For this review, take the finished solid that the model builds, in its own axes (mm). A direction names the side the tool comes from. Give positions to 0.01 mm unless a question says otherwise; leave off trailing zeros. Write each loop counter-clockwise with the first axis right and the second up, starting at its lowest first coordinate (ties: lowest second). Pieces come first, ordered by that corner, then holes. Notation, with made-up numbers: (69.5, -16.75) -> (126.5, -16.75) arc R28 ccw to (126.5, 14.25) -> close; hole circle Ø7 at (45, 7.5). An arc over 180 degrees is marked (long way). Write item = value, one per line.
```python
from build123d import *

# Parameters (mm, degrees)
F0_W     = 76.2
F0_H     = 76.2
F1_DEPTH = 76.2
F2_R     = 11.2668024736
F3_DEPTH = 76.201
F4_W     = 32.2091430426
F4_H     = 35.9837710857
F5_DEPTH = 76.201
F6_R     = 5.08
F7_R     = 5.08


with BuildPart() as f1:
    # F0 (on Top) → F1 (new body)
    with BuildSketch(Plane.XY):
        with Locations((38.1, 38.1)):
            Rectangle(F0_W, F0_H)
    extrude(amount=F1_DEPTH)

    # F2 (on face) → F3 (cut, through all)
    with BuildSketch(Plane.XY.offset(76.2)):
        with Locations((35.9600186348, 40.4836237431)):
            Circle(F2_R)
    extrude(amount=-F3_DEPTH, mode=Mode.SUBTRACT)

    # F4 (on face) → F5 (cut, through all)
    with BuildSketch(Plane.YZ.offset(76.2)):
        with Locations((35.8842462301, 41.1003679037)):
            Rectangle(F4_W, F4_H)
    extrude(amount=-F5_DEPTH, mode=Mode.SUBTRACT)

    # F6
    f6_edges = [f1.edges().sort_by_distance(p)[0] for p in [
        (38.1, 0, 76.2),
        (76.2, 38.1, 76.2),
        (38.1, 76.2, 76.2),
        (0, 38.1, 76.2),
        (0, 0, 38.1),
        (76.2, 0, 38.1),
        (38.1, 0, 0),
        (76.2, 38.1, 0),
        (76.2, 35.884246, 23.108482),
        (76.2, 51.988818, 41.100368),
        (76.2, 76.2, 38.1),
        (76.2, 19.779675, 41.100368),
        (76.2, 35.884246, 59.092253),
        (0, 76.2, 38.1),
        (38.1, 76.2, 0),
        (0, 38.1, 0),
        (24.693216, 40.483624, 0),
    ]]
    fillet(f6_edges, radius=F6_R)

    # F7
    f7_edges = [f1.edges().sort_by_distance(p)[0] for p in [
        (38.1, 5.08, 76.2),
        (5.08, 38.1, 76.2),
        (71.12, 38.1, 76.2),
        (38.1, 71.12, 76.2),
        (24.693216, 40.483624, 76.2),
        (0, 38.1, 71.12),
        (0, 71.12, 38.1),
        (0, 5.08, 38.1),
        (0, 38.1, 5.08),
        (0, 51.988818, 41.100368),
        (0, 35.884246, 59.092253),
        (0, 19.779675, 41.100368),
        (0, 35.884246, 23.108482),
    ]]
    fillet(f7_edges, radius=F7_R)


solid = f1.part
```
(1) Take a section at B-B (x = 18). Write out the cut boundary in (y, z), plus the area to 3 significant figures.
Answers below:
outline = (0, 5.08) arc R5.08 ccw to (5.08, 0) -> (71.12, 0) arc R5.08 ccw to (76.2, 5.08) -> (76.2, 71.12) arc R5.08 ccw to (71.12, 76.2) -> (5.08, 76.2) arc R5.08 ccw to (0, 71.12) -> close; hole (19.78, 23.11) -> (51.99, 23.11) -> (51.99, 59.09) -> (19.78, 59.09) -> close
area = 4,630 mm^2
(2) For pin 1 (13.5 mm diameter, centred on x = 35.96, y = 40.48, fed in from -Z), flat-tipped, find the tip position at first contact; note if it passes through.
Answers below:
pin_1 = through
(3) Take a section at C-C (z = 60.5). Write out the cut boundary in (x, y), plus the area to 3 significant figures.
Answers below:
outline = (0, 5.08) arc R5.08 ccw to (5.08, 0) -> (71.12, 0) arc R5.08 ccw to (76.2, 5.08) -> (76.2, 14.7) arc R5.08 ccw to (74.63, 18.37) -> (74.63, 53.4) arc R5.08 ccw to (76.2, 57.07) -> (76.2, 71.12) arc R5.08 ccw to (71.12, 76.2) -> (5.08, 76.2) arc R5.08 ccw to (0, 71.12) -> (0, 57.07) arc R5.08 ccw to (1.57, 53.4) -> (1.57, 18.37) arc R5.08 ccw to (0, 14.7) -> close; hole circle Ø22.53 at (35.96, 40.48)
area = 5,270 mm^2
(4) Take a section at D-D (z = 12). Write out the cut boundary in (x, y).
Answers below:
outline = (0, 5.08) arc R5.08 ccw to (5.08, 0) -> (71.12, 0) arc R5.08 ccw to (76.2, 5.08) -> (76.2, 71.12) arc R5.08 ccw to (71.12, 76.2) -> (5.08, 76.2) arc R5.08 ccw to (0, 71.12) -> close; hole circle Ø22.53 at (35.96, 40.48)
(5) The part is to be moulded in two halves that separate along Y. For faces 4 (the face through (74.672, 38.562, 1.449)), 5 (the face through (39, 29, 59.092)), 6 (the face through (1.449, 74.672, 38.562)), say which applies: released by +Y, released by -Y, zero draft, split by the parting line, or undercut.
Answers below:
face_4 = zero draft
face_5 = undercut
face_6 = released by +Y
(6) Tool access review of faces 1 (the face through (74.672, 18.331, 41.423)), 2 (the face through (39, 51.989, 41)), 3 (the face through (1.45, 35.59, 21.58)): name each direction out of +Z, -Z, +X, -X, +Y, -Y from which nothing blocks a thin tool from reaching the whole face with its end or side.
Answers below:
face_1 = +X
face_2 = +X, -X
face_3 = -X
(7) Take a section at A-A (z = 36). Write out the cut boundary in (x, y), plus the area to 3 significant figures.
Answers below:
outline = (0, 5.08) arc R5.08 ccw to (5.08, 0) -> (71.12, 0) arc R5.08 ccw to (76.2, 5.08) -> (76.2, 14.7) arc R5.08 ccw to (71.12, 19.78) -> (5.08, 19.78) arc R5.08 ccw to (0, 14.7) -> close; (0, 57.07) arc R5.08 ccw to (5.08, 51.99) -> (71.12, 51.99) arc R5.08 ccw to (76.2, 57.07) -> (76.2, 71.12) arc R5.08 ccw to (71.12, 76.2) -> (5.08, 76.2) arc R5.08 ccw to (0, 71.12) -> close
area = 3,310 mm^2
(8) To check wall thickness, follow probe 1 along Z at (x, y) = (69.5, 44); probe 2 along Y at (x, z) = (52.5, 42.5); probe 3 along Z at (x, y) = (25, 46.5). State the ranges of each line that lie inside material, in increasing order.
Answers below:
probe_1 = 0 to 23.11, 59.09 to 76.2
probe_2 = 0 to 19.78, 51.99 to 76.2
probe_3 = 1.76 to 23.11, 59.09 to 74.44
